Verification items for the finished model (mm, model axes). Face numbers are marked on the shaded views. Round coordinates to 2 decimals unless told otherwise and drop trailing zeros. Write each loop counter-clockwise with the first axis right and the second up, starting at its lowest first coordinate (ties: lowest second). Pieces come first, ordered by that corner, then holes. Notation, with made-up numbers: (-1, 72.5) - (40, 72.5) arc R14 cw to (40, 98.5) - close; hole circle Ø8 at (45.25, 81.5). An arc over 180 degrees is marked (long way). Answer as a JSON object with one key per item and string values.
```python
from build123d import *

# Parameters (mm, degrees)
EXTRUDE005_DEPTH = 3
EXTRUDE006_DEPTH = 3
RECTANGLE001_W   = 100
RECTANGLE001_H   = 100
EXTRUDE004_DEPTH = 50
EXTRUDE007_DEPTH = 3


with BuildPart() as extrude005:
    # Clone2D → Extrude005 (new body)
    with BuildSketch(Plane(origin=(-17, 30, 0), x_dir=(1, 0, 0), z_dir=(0, 0, 1))):
        Polygon((17.44346, -4.685924), (26.023636, -19.546554), (21.745595, -19.546554), (21.745595, -53.769589), (13.140465, -53.769589), (13.140465, -19.546554), (8.861994, -19.546554), align=None)
    extrude(amount=-EXTRUDE005_DEPTH)


with BuildPart() as extrude006:
    # Clone2D001 → Extrude006 (new body)
    with BuildSketch(Plane(origin=(-45, 30, 0), x_dir=(1, 0, 0), z_dir=(0, 0, 1))):
        Polygon((17.44346, -4.685924), (26.023636, -19.546554), (21.745595, -19.546554), (21.745595, -53.769589), (13.140465, -53.769589), (13.140465, -19.546554), (8.861994, -19.546554), align=None)
    extrude(amount=-EXTRUDE006_DEPTH)


with BuildPart() as extrude004:
    # Rectangle001 → Extrude004 (new body)
    with BuildSketch(Plane(origin=(-50, 50, 0), x_dir=(1, 0, 0), z_dir=(0, 0, 1))):
        with Locations((50, -50)):
            Rectangle(RECTANGLE001_W, RECTANGLE001_H)
    extrude(amount=-EXTRUDE004_DEPTH)


with BuildPart() as cut001:
    # Sphere001 → Sphere001 (revolve)
    with BuildSketch(Plane.XZ):
        with BuildLine():
            ThreePointArc((0, -50), (50, 0), (0, 50))
            Line((0, 50), (0, -50))
        make_face()
    revolve(axis=Axis((0, 0, 0), (0, 0, 1)))

    # Cut001: cut Extrude004
    add(extrude004.part, mode=Mode.SUBTRACT)


with BuildPart() as obj1:
    # Clone2D002 → Extrude007 (new body)
    with BuildSketch(Plane(origin=(11, 30, 0), x_dir=(1, 0, 0), z_dir=(0, 0, 1))):
        Polygon((17.44346, -4.685924), (26.023636, -19.546554), (21.745595, -19.546554), (21.745595, -53.769589), (13.140465, -53.769589), (13.140465, -19.546554), (8.861994, -19.546554), align=None)
    extrude(amount=-EXTRUDE007_DEPTH)

    # Fusion003: union Extrude005, Extrude006, Cut001
    add(extrude005.part)
    add(extrude006.part)
    add(cut001.part)


solid = obj1.part
```
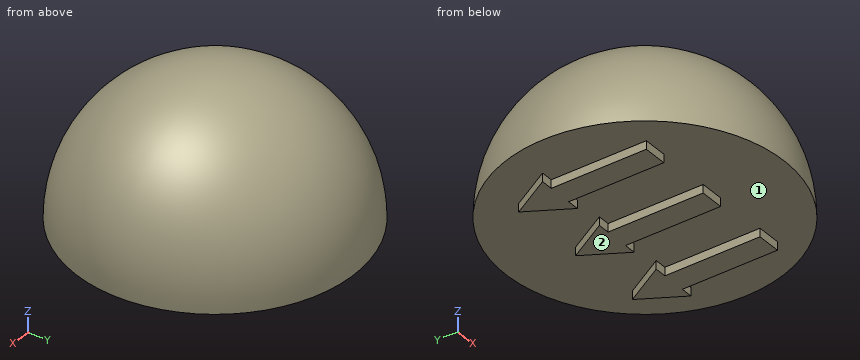
Q1. Section check D-D, the plane y = 21.5. Record the cut outline in (x, z).
Geometry check:
{"outline": "(-45.14, 0) - (-29.76, 0) - (-29.76, -3) - (-25.35, -3) - (-25.35, 0) - (-1.76, 0) - (-1.76, -3) - (2.65, -3) - (2.65, 0) - (26.24, 0) - (26.24, -3) - (30.65, -3) - (30.65, 0) - (45.14, 0) arc R45.14 ccw to start"}
Q2. Release check for a two-part mould opening along X. For the marked faces 1 and 2 record: released by +X, released by -X, zero draft, split by the parting line, or undercut.
Geometry check:
{"face 1": "undercut", "face 2": "zero draft"}
Q3. Section check B-B, the plane x = -42. Record the cut outline in (y, z).
Geometry check:
{"outline": "(-27.13, 0) - (27.13, 0) arc R27.13 ccw to start"}
Q4. Material ranges on line 1 along X through (y, z) = (31, 4); line 2 along Z through (x, y) = (-24.5, -34.5); line 3 along X through (y, z) = (5, 7), recorded low to high. Write a range as [from, to].
Geometry check:
{"line 1": "x = [-39.03, 39.03]", "line 2": "z = [0, 26.64]", "line 3": "x = [-49.25, 49.25]"}
Q5. Section check C-C, the plane z = 13. Record the cut outline in (x, y).
Geometry check:
{"outline": "circle Ø96.56 at (0, 0)"}
Q6. Section check A-A, the plane y = -19.5. Record the cut outline in (x, z).
Geometry check:
{"outline": "(-46.04, 0) - (-31.86, 0) - (-31.86, -3) - (-23.25, -3) - (-23.25, 0) - (-3.86, 0) - (-3.86, -3) - (4.75, -3) - (4.75, 0) - (24.14, 0) - (24.14, -3) - (32.75, -3) - (32.75, 0) - (46.04, 0) arc R46.04 ccw to start"}
Q7. Gauge pin test, flat ends, axial feed: P1, Ø1.5, axis at x = 27, z = -1, coming from the -Y side; P2, Ø10, axis at y = -14.5, z = 29, coming from the +X side; P3, Ø3.5, axis at x = -21, z = -1, coming from the -Y side. Record the tip position at first contact, or that the pin passes through.
Geometry check:
{"P1": "stops at y = -23.77", "P2": "stops at x = 41.81", "P3": "stops at y = -46.01"}
